Drawing for the job (mm, zero at the part's lowest x, y, z). A direction names the side the tool comes from. Round coordinates to 2 decimals unless told otherwise and drop trailing zeros. Loops run counter-clockwise (first coordinate to the right, second up) from the corner with the lowest first, then second, coordinate; pieces in that order, holes last. Notation, with made-up numbers: (33, 74) - (47, 74) arc R33 cw to (47, 109) - close; hole circle Ø10 at (37, 70.25). An arc over 180 degrees is marked (long way). Put each result on its own line as item: value.
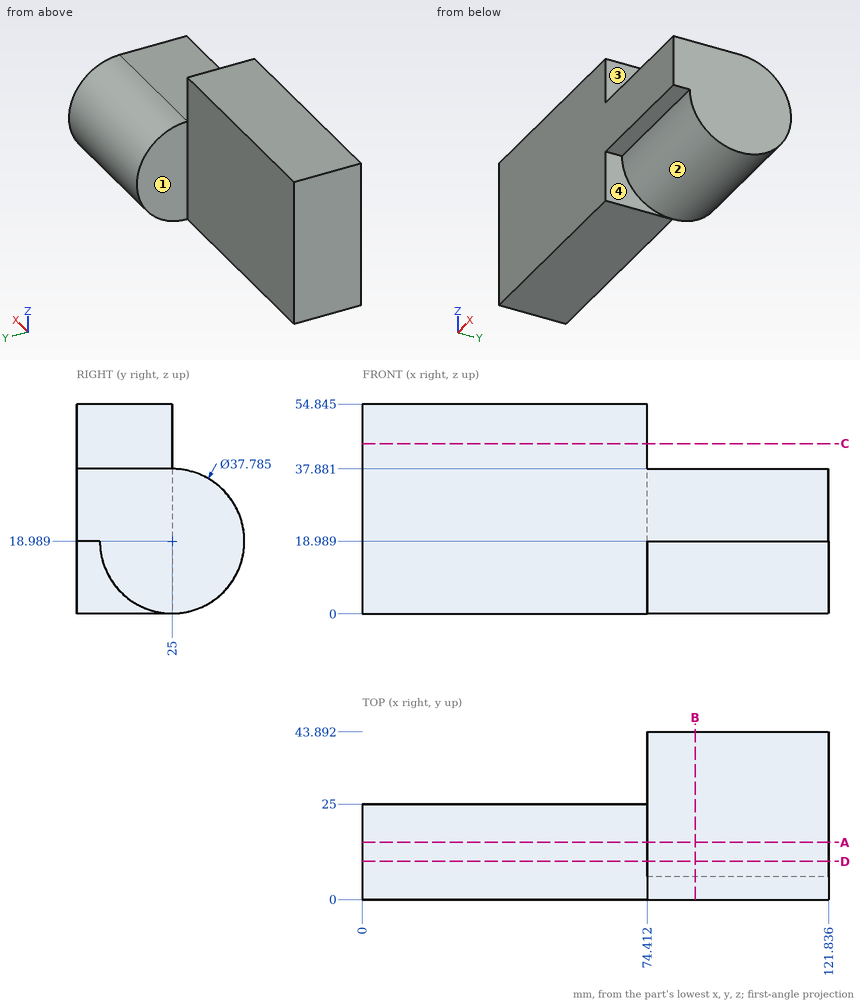
1. Pin check, flat tips, straight feed: P1, Ø5, axis at x = 90.5, y = 18, coming from the +Z side; P2, Ø2, axis at x = 103, y = 36, coming from the -Z side; P3, Ø16.5, axis at x = 54.5, z = 14, coming from the +Y side. Stop position of each tip, or through.
A:
P1: stops at z = 37.88
P2: stops at z = 2.96
P3: stops at y = 25
2. Band-saw the part on B-B (x = 87). List the corners of the cut face in (y, z) (1 decimal).
A:
outline: (0, 19) - (6.1, 19) arc R18.9 ccw (long way) to (25, 37.9) - (0, 37.9) - close
3. Band-saw the part on D-D (y = 10). List the corners of the cut face in (x, z) (1 decimal), plus the area to 3 significant figures.
A:
outline: (0, 0) - (74.4, 0) - (74.4, 7.5) - (121.8, 7.5) - (121.8, 37.9) - (74.4, 37.9) - (74.4, 54.8) - (0, 54.8) - close
area: 5,520 mm²
4. Band-saw the part on C-C (z = 44.5). List the corners of the cut face in (x, y).
A:
outline: (0, 0) - (74.41, 0) - (74.41, 25) - (0, 25) - close
5. Probe line 1 along Y through (x, z) = (57, 13.5); line 2 along X through (y, z) = (27.5, 37); line 3 along X through (y, z) = (22.5, 43). List the from-to ranges inside material, lowest first. Write a range as [from, to].
A:
line 1: y = [0, 25]
line 2: x = [74.41, 121.84]
line 3: x = [0, 74.41]
6. Tool access for the marked faces 1, 2, 3 and 4: list every direction of +Z, -Z, +X, -X, +Y, -Y with a clear straight run to the whole face (end or side of a thin tool).
A:
face 1: +Z, -Z, -X, +Y
face 2: +X
face 3: +Z, +X, +Y, -Y
face 4: -Z, +X, -Y
7. Band-saw the part on A-A (y = 15). List the corners of the cut face in (x, z) (1 decimal), plus the area to 3 significant figures.
A:
outline: (0, 0) - (74.4, 0) - (74.4, 3) - (121.8, 3) - (121.8, 37.9) - (74.4, 37.9) - (74.4, 54.8) - (0, 54.8) - close
area: 5,740 mm²
